Here's the drawing with two shaded views (mm, measured from the low corner). I have some questions. Give positions to 0.01 mm unless a question says otherwise; leave off trailing zeros. Loops run counter-clockwise (first coordinate to the right, second up) from the corner with the lowest first, then second, coordinate; pieces in that order, holes last. Notation, with made-up numbers: (50, 82.25) - (92, 82.25) arc R25 ccw to (92, 113.25) - close; hole circle Ø1 at (15.5, 35.25). An arc over 180 degrees is marked (long way). Use one line per item in the form item = value.
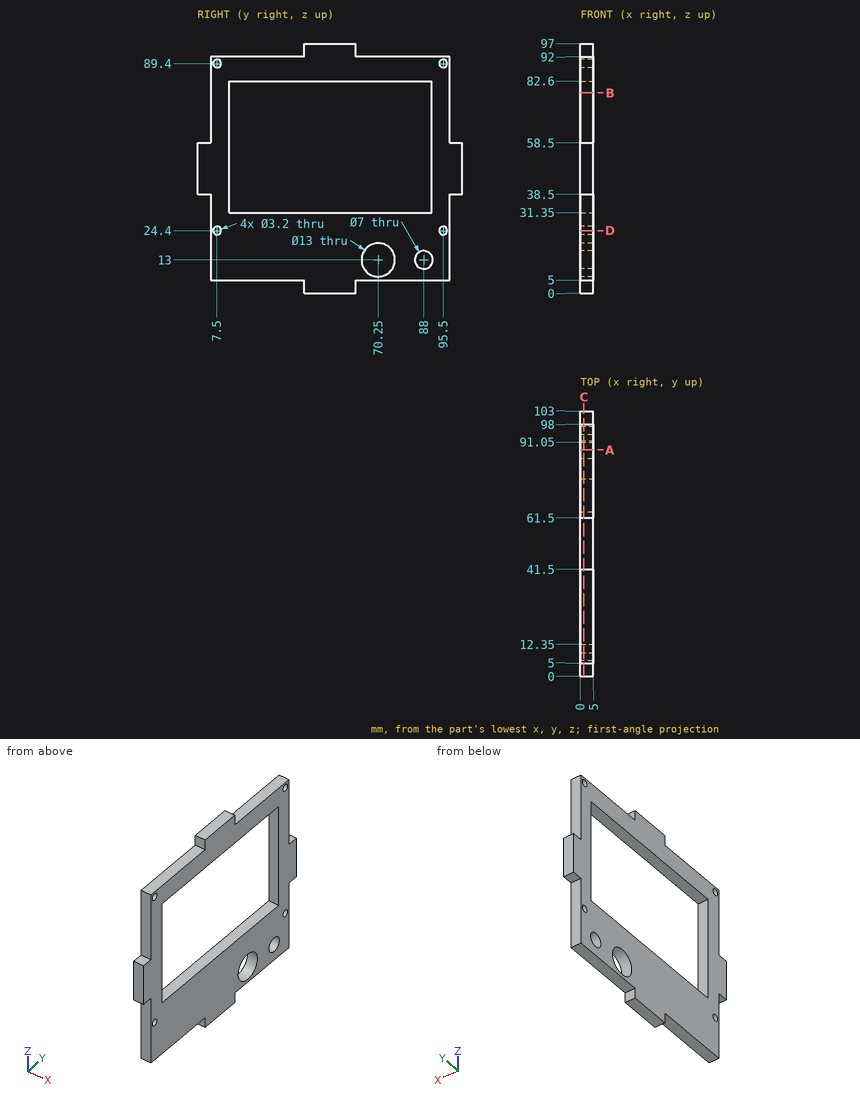
(1) If we section it at D-D (z = 24.4): List the corners of the cut face in (x, y) for me, plus the area to 3 significant figures.
Geometry says:
outline = (0, 5) - (5, 5) - (5, 5.9) - (0, 5.9) - close; (0, 9.1) - (5, 9.1) - (5, 93.9) - (0, 93.9) - close; (0, 97.1) - (5, 97.1) - (5, 98) - (0, 98) - close
area = 433 mm²
(2) If we section it at A-A (y = 88): List the corners of the cut face in (x, z) for me, plus the area to 3 significant figures.
Geometry says:
outline = (0, 5) - (5, 5) - (5, 9.5) - (0, 9.5) - close; (0, 16.5) - (5, 16.5) - (5, 31.35) - (0, 31.35) - close; (0, 82.6) - (5, 82.6) - (5, 92) - (0, 92) - close
area = 144 mm²
(3) If we section it at B-B (z = 78): List the corners of the cut face in (x, y) for me, plus the area to 3 significant figures.
Geometry says:
outline = (0, 5) - (5, 5) - (5, 12.35) - (0, 12.35) - close; (0, 91.05) - (5, 91.05) - (5, 98) - (0, 98) - close
area = 71.5 mm²
(4) If we section it at C-C (x = 1.3): Give the number of separate pieces and of enclosed holes in the cut face, plus the area to 3 significant figures.
Geometry says:
separate_pieces = 1
enclosed_holes = 7
area = 4,250 mm²
(5) For P1, Ø2.5, axis at x = 1.5, z = 94.5, coming from the +Y side; P2, Ø3, axis at x = 1, z = 79, coming from the +Y side; P3, Ø1.5, axis at x = 2.5, y = 100, coming from the -Z side, each with a flat end and sliding along its axis, tell me the tip position at first contact or that it passes through.
Geometry says:
P1 = 61.5
P2 = 98
P3 = 38.5
(6) If I drill on probe 1 along Z at (x, y) = (1.1, 70); probe 2 along Y at (x, z) = (1.85, 89.4); probe 3 along Z at (x, y) = (3.35, 7.5), over which ranges is the centre line in solid material (lowest first)?
Geometry says:
probe_1 = 5 to 6.5, 19.5 to 31.35, 82.6 to 92
probe_2 = 5 to 5.9, 9.1 to 93.9, 97.1 to 98
probe_3 = 5 to 22.8, 26 to 87.8, 91 to 92
